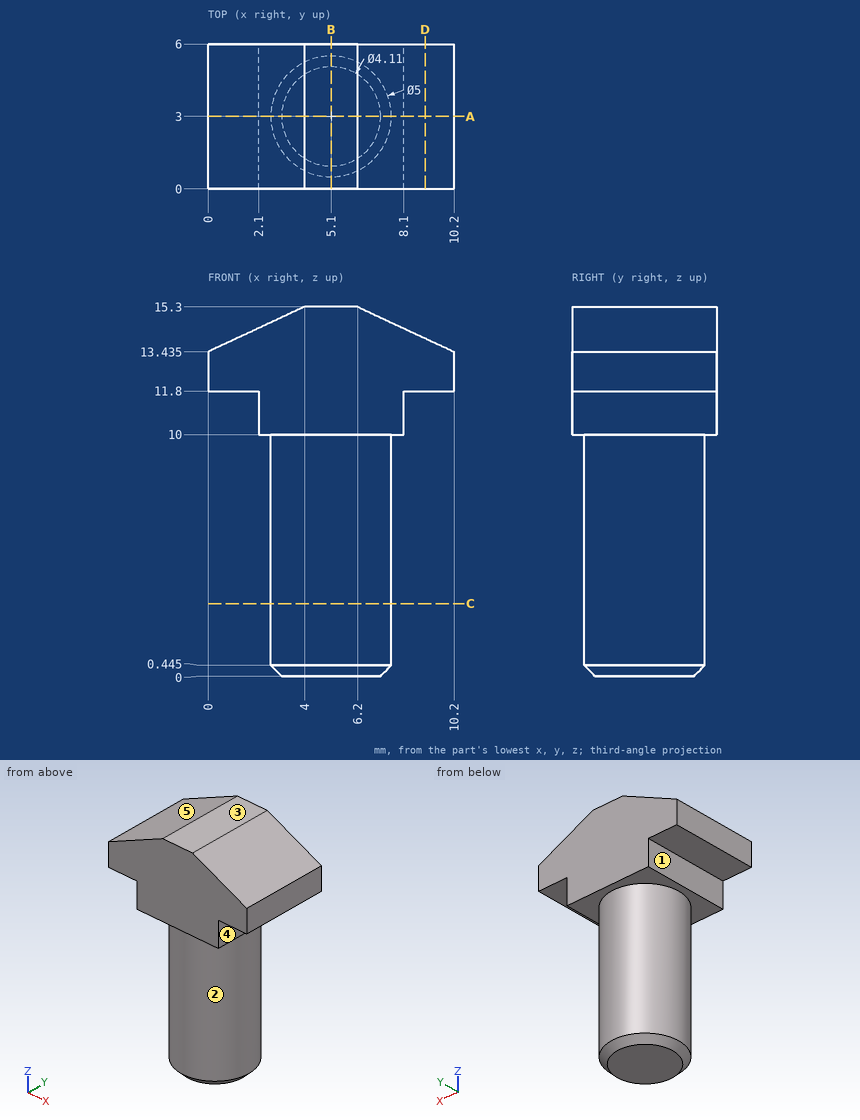
Print and shaded views of the part. All mm, measured from the part's lowest x, y and z. A direction names the side the tool comes from. Round coordinates to 2 decimals unless told otherwise and drop trailing zeros. Order: outer loops, then holes, each group sorted by start corner. A loop starts at its lowest first (then second) coordinate and runs counter-clockwise, first axis right, second up.
Q1. Drop flat-ended pins along their axis: pin 1 (1 mm diameter, centred on x = 3, y = 5, fed in from +Z); pin 2 (0.6 mm diameter, centred on x = 1.5, y = 2, fed in from -Z); pin 3 (2 mm diameter, centred on y = 1.5, z = 9.5, fed in from +X). Give the stop position or say it passes through.
Q2. Slice it at D-D (x = 9). Write the cut outline in (y, z), and give its area (3 significant figures).
Q3. Slice it at C-C (z = 3). Write the cut outline in (x, y), and give its area (3 significant figures).
Q4. Wall check: L1, parallel to X at y = 1.7, z = 10.25; L2, parallel to Z at x = 7, y = 2; L3, parallel to Y at x = 3.5, z = 6. Give the ranges that are in metal, low to high.
Q5. Slice it at A-A (y = 3). Write the cut outline in (x, z) (1 decimal).
Q6. Which spindle directions (+Z, -Z, +X, -X, +Y, -Y) get a long thin tool onto all of the face, cutting with end or side? Do the marked faces 1, 2, 3, 4 and 5. Say none if no direction does.
Q7. Slice it at B-B (x = 5.1). Write the cut outline in (y, z) (3 decimals).
Results below:
1. pin 1: stops at z = 15.07
1. pin 2: stops at z = 11.8
1. pin 3: stops at x = 8.1
2. outline: (0, 11.8) - (6, 11.8) - (6, 13.99) - (0, 13.99) - close
2. area: 13.2 mm2
3. outline: circle Ø5 at (5.1, 3)
3. area: 19.6 mm2
4. L1: x = 2.1 to 8.1
4. L2: z = 0.09 to 14.93
4. L3: y = 1.08 to 4.92
5. outline: (0, 11.8) - (2.1, 11.8) - (2.1, 10) - (2.6, 10) - (2.6, 0.4) - (3, 0) - (7.2, 0) - (7.6, 0.4) - (7.6, 10) - (8.1, 10) - (8.1, 11.8) - (10.2, 11.8) - (10.2, 13.4) - (6.2, 15.3) - (4, 15.3) - (0, 13.4) - close
6. face 1: -Z, -X, +Y, -Y
6. face 2: -Z
6. face 3: +Z, +X, -X, +Y, -Y
6. face 4: -Z, +X, +Y, -Y
6. face 5: +Z, -X, +Y, -Y
7. outline: (0, 10) - (0.5, 10) - (0.5, 0.445) - (0.945, 0) - (5.055, 0) - (5.5, 0.445) - (5.5, 10) - (6, 10) - (6, 15.3) - (0, 15.3) - close
